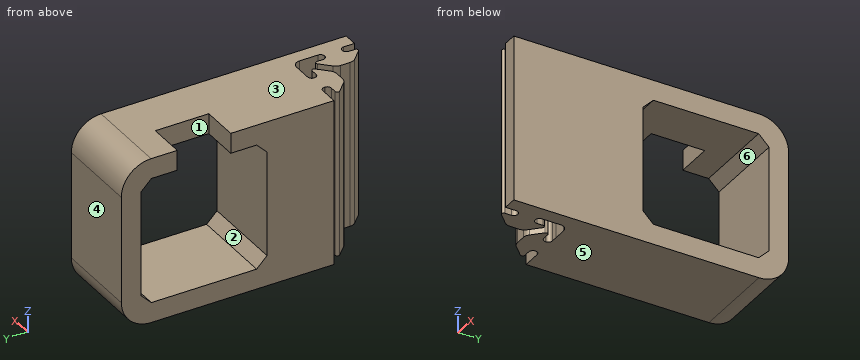
```python
from build123d import *

# Parameters (mm, degrees)
BOSS_EXTRUDE1_DEPTH = 56
SKETCH14_W          = 42.4
SKETCH14_H          = 42.4
CUT_EXTRUDE1_DEPTH  = 56
CHAMFER1_SIZE       = 3.5
FILLET1_R           = 10
CUT_EXTRUDE4_REACH  = 104.922
SKETCH17_W          = 15.453545708
SKETCH17_H          = 18


with BuildPart() as part:
    # Sketch1 → Boss-Extrude1 (new body)
    with BuildSketch(Plane.XY):
        with BuildLine():
            Line((13.02, -7.9417418), (17.7, -7.9417418))
            Line((17.7, -7.9417418), (17.7, 84.52))
            Line((17.7, 84.52), (-10.566443095, 84.52))
            Line((-10.566443095, 84.52), (-10.566443095, 13.02))
            Line((-10.566443095, 13.02), (-5.317126718, 13.02))
            Line((-5.317126718, 13.02), (-4.287512407, 13.02))
            ThreePointArc((-4.287512407, 13.02), (-3.319474451, 12.619025549), (-2.9185, 11.650987593))
            Line((-2.9185, 11.650987593), (-2.9185, 11.539212407))
            ThreePointArc((-2.9185, 11.539212407), (-3.319474451, 10.571174451), (-4.287512407, 10.1702))
            Line((-4.287512407, 10.1702), (-6.476788598, 10.1702))
            ThreePointArc((-6.476788598, 10.1702), (-7.136510935, 9.729114651), (-6.981020848, 8.950903446))
            Line((-6.981020848, 8.950903446), (-3.672257405, 5.649701928))
            ThreePointArc((-3.672257405, 5.649701928), (-2.746830644, 5.032499411), (-1.655778399, 4.8158))
            Line((-1.655778399, 4.8158), (1.655778399, 4.8158))
            ThreePointArc((1.655778399, 4.8158), (2.746830644, 5.032499411), (3.672257405, 5.649701928))
            Line((3.672257405, 5.649701928), (6.981020848, 8.950903446))
            ThreePointArc((6.981020848, 8.950903446), (7.136510935, 9.729114651), (6.476788598, 10.1702))
            Line((6.476788598, 10.1702), (4.287512407, 10.1702))
            ThreePointArc((4.287512407, 10.1702), (3.319474451, 10.571174451), (2.9185, 11.539212407))
            Line((2.9185, 11.539212407), (2.9185, 11.650987593))
            ThreePointArc((2.9185, 11.650987593), (3.319474451, 12.619025549), (4.287512407, 13.02))
            Line((4.287512407, 13.02), (6.332886163, 13.02))
            Line((6.332886163, 13.02), (10.562594215, 13.019824354))
            ThreePointArc((10.562594215, 13.019824354), (12.303594776, 12.313982883), (13.019956614, 10.577284622))
            Line((13.019956614, 10.577284622), (13.02, 4.287469289))
            ThreePointArc((13.02, 4.287469289), (12.619025549, 3.319431332), (11.650987593, 2.918456882))
            Line((11.650987593, 2.918456882), (11.539212407, 2.918456882))
            ThreePointArc((11.539212407, 2.918456882), (10.571174451, 3.319431332), (10.1702, 4.287469289))
            Line((10.1702, 4.287469289), (10.1702, 6.402089023))
            ThreePointArc((10.1702, 6.402089023), (9.733877283, 7.055496588), (8.963146507, 6.90287605))
            Line((8.963146507, 6.90287605), (5.667020993, 3.614283579))
            ThreePointArc((5.667020993, 3.614283579), (5.046449321, 2.687255303), (4.8285, 1.593185507))
            Line((4.8285, 1.593185507), (4.8285, -1.593185507))
            ThreePointArc((4.8285, -1.593185507), (5.046449321, -2.687255303), (5.667020993, -3.614283579))
            Line((5.667020993, -3.614283579), (8.963146507, -6.90287605))
            ThreePointArc((8.963146507, -6.90287605), (9.733877283, -7.055496588), (10.1702, -6.402089023))
            Line((10.1702, -6.402089023), (10.1702, -4.287469289))
            ThreePointArc((10.1702, -4.287469289), (10.571174451, -3.319431332), (11.539212407, -2.918456882))
            Line((11.539212407, -2.918456882), (11.650987593, -2.918456882))
            ThreePointArc((11.650987593, -2.918456882), (12.619025549, -3.319431332), (13.02, -4.287469289))
            Line((13.02, -4.287469289), (13.02, -5.3170836))
            Line((13.02, -5.3170836), (13.02, -7.9417418))
        make_face()
    extrude(amount=BOSS_EXTRUDE1_DEPTH)

    # Sketch14 → Cut-Extrude1 (cut)
    with BuildSketch(Plane(origin=(17.7, 0, 0), x_dir=(0, 0, -1), z_dir=(1, 0, 0))):
        with Locations((-28, 56.72)):
            Rectangle(SKETCH14_W, SKETCH14_H)
    extrude(amount=-CUT_EXTRUDE1_DEPTH, mode=Mode.SUBTRACT)

    # Chamfer1
    chamfer1_edges = [part.edges().sort_by_distance(p)[0] for p in [
        (3.566778452, 35.52, 49.2),
        (3.566778452, 77.92, 49.2),
        (3.566778452, 77.92, 6.8),
        (3.566778452, 35.52, 6.8),
    ]]
    chamfer(chamfer1_edges, length=CHAMFER1_SIZE)

    # Fillet1
    fillet1_edges = [part.edges().sort_by_distance(p)[0] for p in [
        (3.566778452, 84.52, 56),
        (3.566778452, 84.52, 0),
    ]]
    fillet(fillet1_edges, radius=FILLET1_R)

    # Sketch17 → Cut-Extrude4 (cut, up to next)
    with BuildSketch(Plane.XY.offset(56), mode=Mode.PRIVATE) as cut_extrude4_sk1:
        with Locations((-5.893215949, 56.72)):
            Rectangle(SKETCH17_W, SKETCH17_H)
    cut_extrude4_tool1 = extrude(cut_extrude4_sk1.sketch, amount=-CUT_EXTRUDE4_REACH, mode=Mode.PRIVATE) & part.part
    add(cut_extrude4_tool1.solids().sort_by_distance((-5.893216, 56.72, 56))[0], mode=Mode.SUBTRACT)


solid = part.part
```
Part model, mm, in its own coordinate system. Face numbers are marked on the shaded views. A direction names the side the tool comes from. Round coordinates to 2 decimals unless told otherwise and drop trailing zeros. Order: outer loops, then holes, each group sorted by start corner. A loop starts at its lowest first (then second) coordinate and runs counter-clockwise, first axis right, second up. Notation, with made-up numbers: M -31.75,59 L 24.25,59 A14 ccw 24.25,66 Z; hole C -25.75,-32 d11. An arc over 180 degrees is marked long. Answer in a Markdown table with one row per item. Add a question column.
Q1. Cut at B-B on x = -5.25. Give the cut face in (y, z), and give its area (3 significant figures).
Q2. Mould opens along Y. For the marked faces 4, 5 and 6 say: +Y half, -Y half, draft (parallel to the pull), parting line (faces both ways), or undercut.
Q3. Wall check: L1, parallel to Z at x = 6.5, y = 67; L2, parallel to Y at x = -1, z = 31.5; L3, parallel to Y at x = 10.5, z = 25.5. Give the ranges that are in metal, low to high. Write a range as from..to.
Q4. Pin check, flat tips, straight feed: pin 1 (7.5 mm diameter, centred on x = -5, z = 51.5, fed in from -Y); pin 2 (5.5 mm diameter, centred on y = 54.5, z = 52.5, fed in from -X); pin 3 (2 mm diameter, centred on x = 5.5, z = 35.5, fed in from -Y). Stop position of each tip, or through.
Q5. Cut at A-A on y = 59.5. Give the cut face in (x, z), and give its area (3 significant figures).
Q6. 3-axis set-ups, long thin cutter, end or side, ignore diameter. For the marked faces 1, 2 and 3: which of +Z, -Z, +X, -X, +Y, -Y reach the whole face in a straight line?
Established:
| question | item | result |
|---|---|---|
| 1 | outline | M 7.22,0 L 10.17,0 L 10.17,56 L 7.22,56 Z; M 13.02,0 L 74.52,0 A10 ccw 84.52,10 L 84.52,46 A10 ccw 74.52,56 L 65.72,56 L 65.72,49.2 L 74.42,49.2 L 77.92,45.7 L 77.92,10.3 L 74.42,6.8 L 39.02,6.8 L 35.52,10.3 L 35.52,45.7 L 39.02,49.2 L 47.72,49.2 L 47.72,56 L 13.02,56 Z |
| 1 | area | 2,230 mm2 |
| 2 | face 4 | +Y half |
| 2 | face 5 | draft |
| 2 | face 6 | undercut |
| 3 | L1 | z = 0..6.8, 49.2..56 |
| 3 | L2 | y = 4.82..35.52, 77.92..84.52 |
| 3 | L3 | y = -3.4..3.4, 13.02..35.52, 77.92..84.52 |
| 4 | pin 1 | stops at y = 4.82 |
| 4 | pin 2 | stops at x = 1.83 |
| 4 | pin 3 | stops at y = -4.45 |
| 5 | outline | M -10.57,0 L 17.7,0 L 17.7,6.8 L -10.57,6.8 Z; M 1.83,49.2 L 17.7,49.2 L 17.7,56 L 1.83,56 Z |
| 5 | area | 300 mm2 |
| 6 | face 1 | +Z, -X |
| 6 | face 2 | +X, -X |
| 6 | face 3 | +Z, +X, -X, +Y, -Y |
